Job drawing, mm, ordinate dimensions from the low corner. One solid piece. A direction names the side the tool comes from. Give positions to 0.01 mm unless a question says otherwise; leave off trailing zeros. Order: outer loops, then holes, each group sorted by start corner. A loop starts at its lowest first (then second) coordinate and runs counter-clockwise, first axis right, second up.
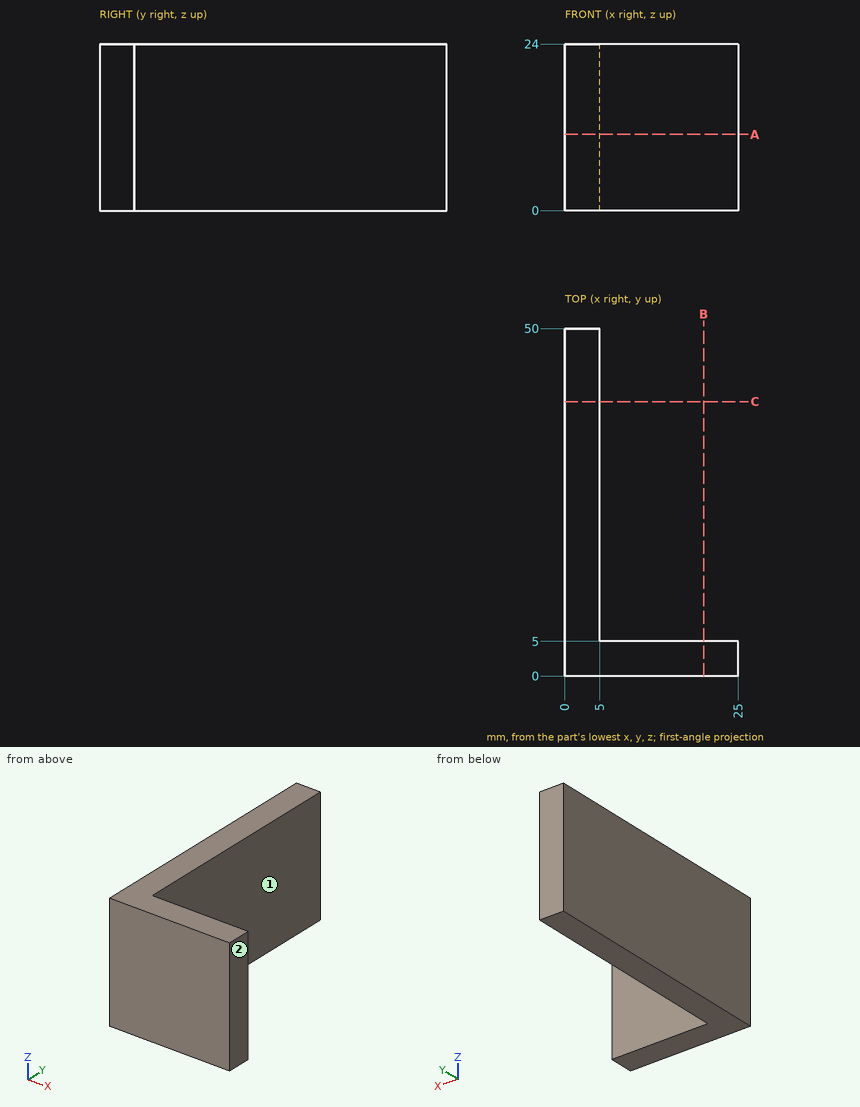
Item 1: Drill centre line: probe 1 along X at (y, z) = (36, 1.5). Where is it in solid material? Low to high.
Item 2: Band-saw the part on B-B on x = 20. List the corners of the cut face in (y, z), plus the area to 3 significant figures.
Item 3: Band-saw the part on A-A on z = 11. List the corners of the cut face in (x, y).
Item 4: Drop flat-ended pins along their axis: P1, Ø4, axis at y = 28.5, z = 17.5, coming from the +X side; P2, Ø2, axis at x = 20.5, z = 12, coming from the +Y side. Give the stop position or say it passes through.
Item 5: Which spindle directions (+Z, -Z, +X, -X, +Y, -Y) get a long thin tool onto all of the face, cutting with end or side? Do the marked faces 1 and 2. Say none if no direction does.
Working result:
1. probe 1: x = 0 to 5
2. outline: (0, 0) - (5, 0) - (5, 24) - (0, 24) - close
2. area: 120 mm2
3. outline: (0, 0) - (25, 0) - (25, 5) - (5, 5) - (5, 50) - (0, 50) - close
4. P1: stops at x = 5
4. P2: stops at y = 5
5. face 1: +Z, -Z, +X, +Y
5. face 2: +Z, -Z, +X, +Y, -Y
